Verification items for the finished model (mm, model axes). Face numbers are marked on the shaded views. A direction names the side the tool comes from. Round coordinates to 2 decimals unless told otherwise and drop trailing zeros. Order: outer loops, then holes, each group sorted by start corner. A loop starts at its lowest first (then second) coordinate and runs counter-clockwise, first axis right, second up. Notation, with made-up numbers: M 20,-0.75 L 62,-0.75 A24 ccw 62,11.25 Z; hole C 24,35.5 d10. An arc over 180 degrees is marked long. Use one line per item in the form item = value. Start each with the question number.
Item 1: Release check for a two-part mould opening along Z. For the marked faces 1, 2 and 3 record: +Z half, -Z half, draft (parallel to the pull), parting line (faces both ways), or undercut.
Item 2: Tool access check on the marked faces 4 and 5. Record the directions out of +Z, -Z, +X, -X, +Y, -Y that give a thin tool (end or side, any length) a straight path to the whole face; none if there is none.
Item 3: Thickness scan on probe 1 along Y at (x, z) = (35, -0.25); probe 2 along Z at (x, y) = (23, -3.5); probe 3 along Y at (x, z) = (16, -1.75). Record the ranges inside material, lowest first. Write a range as [from, to].
Item 4: Cross-section at A-A on x = 19.5. Enter the section's corners in (y, z), then the cut area to 3 significant figures.
Item 5: Go/stop test with flat-tipped pins: pin 1 Ø2 at (y, z) = (5.5, 1.5) entering from -X; pin 2 Ø0.6 at (y, z) = (-2.5, 0) entering from -X; pin 3 Ø3 at (x, y) = (2, 0.5) entering from -Z. Record where each tip stops, or that it passes through.
from build123d import *

# Parameters (mm, degrees)
FILLET1_R   = 0.4
HEX_2_DEPTH = 2.6


with BuildPart() as part:
    # BodySke → BaseBody (revolve)
    with BuildSketch(Plane.XY, mode=Mode.PRIVATE) as basebody_sk:
        with BuildLine():
            Line((39.4, 0), (39.4, 3.3095))
            Line((39.4, 3.3095), (38.7095, 4))
            Line((38.7095, 4), (4.4, 4))
            Line((4.4, 4), (4.4, 7))
            Line((4.4, 7), (4.02, 7))
            ThreePointArc((4.02, 7), (1.686451133, 5.621618984), (0, 3.5))
            Line((0, 3.5), (0, 0))
            Line((0, 0), (39.4, 0))
        make_face()
    revolve(basebody_sk.sketch.rotate(Axis((0, 0, 0), (1, 0, 0)), 90), axis=Axis((0, 0, 0), (1, 0, 0)))

    # Fillet1
    fillet1_edges = [part.edges().sort_by_distance(p)[0] for p in [
        (4.4, 0, -4),
    ]]
    fillet(fillet1_edges, radius=FILLET1_R)

    # Sketch2 → PreBroach (revolve, cut)
    with BuildSketch(Plane.XY, mode=Mode.PRIVATE) as prebroach_sk:
        Polygon((0, 2.5), (2.6, 2.5), (4.043375673, 0), (0, 0), align=None)
    revolve(prebroach_sk.sketch.rotate(Axis((0, 0, 0), (1, 0, 0)), 90), axis=Axis((0, 0, 0), (1, 0, 0)), mode=Mode.SUBTRACT)

    # Sketch3 → Hex 2 (cut)
    with BuildSketch(Plane(origin=(0, 0, 0), x_dir=(0, 0, -1), z_dir=(1, 0, 0))):
        Polygon((-2.5, -1.443375673), (-2.5, 1.443375673), (0, 2.886751346), (2.5, 1.443375673), (2.5, -1.443375673), (0, -2.886751346), align=None)
    extrude(amount=HEX_2_DEPTH, mode=Mode.SUBTRACT)


solid = part.part
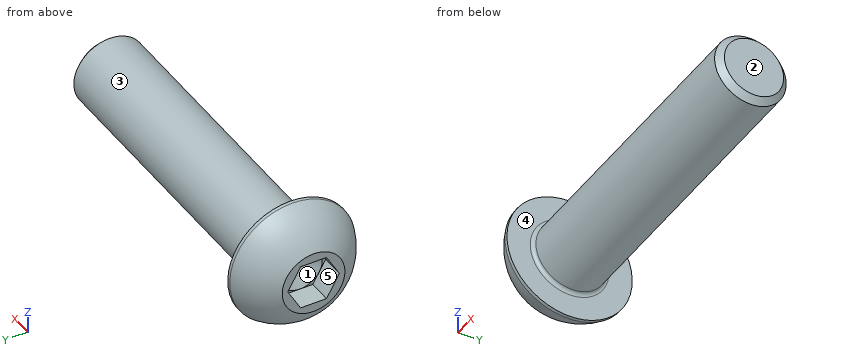
Output values:
q1.face_1 = undercut
q1.face_2 = draft
q1.face_3 = parting line
q2.face_4 = +X
q2.face_5 = -X
q3.probe_1 = [-3.99, 3.99]
q3.probe_2 = [-1.94, 1.94]
q3.probe_3 = [-3.6, 3.6]
q4.outline = C 0,0 d8
q4.area = 50.3 mm2
q5.pin_1 = 0.8
q5.pin_2 = 2.6
q5.pin_3 = -6.77
